Geometry check sheet. Reference: the model listing, model coordinates, mm. A direction names the side the tool comes from. Give positions to 0.01 mm unless a question says otherwise; leave off trailing zeros. Write each loop counter-clockwise with the first axis right and the second up, starting at its lowest first coordinate (ties: lowest second). Pieces come first, ordered by that corner, then holes. Notation, with made-up numbers: (72, 20.25) - (127, 20.25) arc R31 cw to (127, 45.25) - close; hole circle Ø11 at (22, -10.75). An arc over 180 degrees is marked (long way). One line per question, with ' | ' between items. Start each with the question number.
Q1. Release check for a two-part mould opening along X. For faces 1 (the face through (1.802, -72.712, 5.723)), 2 (the face through (4, -219, -4)), 3 (the face through (-209.84, 50.49, 160.9)) record: +X half, -X half, draft (parallel to the pull), parting line (faces both ways), or undercut.
Q2. Thickness scan on L1, parallel to X at y = -75.5, z = 0; L2, parallel to X at y = -131, z = 0; L3, parallel to X at y = 31, z = 112. Record the ranges inside material, lowest first. Write a range as [from, to].
Q3. Section check A-A on y = -139. Record the boundary of the cut face in (x, z), and give its area (3 significant figures).
Q4. Gauge pin test, flat ends, axial feed: P1, Ø6, axis at x = -88.5, y = -6, coming from the -Z side; P2, Ø10, axis at x = 107, z = 54.5, coming from the -Y side; P3, Ø1.5, axis at x = -139, y = -86, coming from the -Z side. Record the tip position at first contact, or that the pin passes through.
Q5. Set-up check for faces 4 (the face through (1.802, -209.321, 5.723)), 5 (the face through (-4, 50, 55)), 6 (the face through (-4, 51, 55)): record each of +Z, -Z, +X, -X, +Y, -Y from which the full face is reachable in a straight line by a thin tool's end or side.
```python
from build123d import *

# Parameters (mm, degrees)
FILLET1_R           = 20
SHELL1_T            = -1
SKETCH3_R           = 264.42717426
BOSS_EXTRUDE1_DEPTH = 1
SKETCH4_R           = 5
CUT_EXTRUDE1_DEPTH  = 451.38257191
SKETCH6_R           = 6
SKETCH6_R_2         = 5
BOSS_EXTRUDE2_DEPTH = 270
FILLET2_R           = 1


with BuildPart() as part:
    # Sketch2 → Revolve1 (revolve)
    with BuildSketch(Plane.XY):
        with BuildLine():
            Line((0, 50), (0, -200))
            ThreePointArc((0, -200), (141.421356237, -141.421356237), (200, 0))
            ThreePointArc((200, 0), (233.555453903, 23.270946312), (264.42717426, 50))
            Line((264.42717426, 50), (0, 50))
        make_face()
    revolve(axis=Axis((0, 50, 0), (0, -1, 0)))

    # Fillet1
    fillet1_edges = [part.edges().sort_by_distance(p)[0] for p in [
        (-200, 0, 0),
    ]]
    fillet(fillet1_edges, radius=FILLET1_R)

    # Shell1
    shell1_openings = [part.faces().sort_by_distance(p)[0] for p in [
        (0, 50, 0),
    ]]
    offset(amount=SHELL1_T, openings=shell1_openings, kind=Kind.INTERSECTION)

    # Sketch3 → Boss-Extrude1 (add)
    with BuildSketch(Plane(origin=(0, 50, 0), x_dir=(1, 0, 0), z_dir=(0, 1, 0))):
        Circle(SKETCH3_R)
    extrude(amount=BOSS_EXTRUDE1_DEPTH)

    # Sketch4 → Cut-Extrude1 (cut, through all)
    with BuildSketch(Plane(origin=(0, 51, 0), x_dir=(1, 0, 0), z_dir=(0, 1, 0))):
        with Locations(Location((0, 0, 0), (0, 0, 270))):
            Circle(SKETCH4_R)
    extrude(amount=-CUT_EXTRUDE1_DEPTH, mode=Mode.SUBTRACT)

    # Sketch6 → Boss-Extrude2 (add)
    with BuildSketch(Plane(origin=(0, 51, 0), x_dir=(1, 0, 0), z_dir=(0, 1, 0))):
        with Locations(Location((0, 0, 0), (0, 0, 270))):
            Circle(SKETCH6_R)
        with Locations(Location((0, 0, 0), (0, 0, 270))):
            Circle(SKETCH6_R_2, mode=Mode.SUBTRACT)
    extrude(amount=-BOSS_EXTRUDE2_DEPTH)

    # Fillet2
    fillet2_edges = [part.edges().sort_by_distance(p)[0] for p in [
        (0, 51, -5),
    ]]
    fillet(fillet2_edges, radius=FILLET2_R)


solid = part.part
```
Working result:
1) face 1: undercut | face 2: draft | face 3: parting line
2) L1: x = [-185.2, -184.12], [-6, -5], [5, 6], [184.12, 185.2] | L2: x = [-151.13, -149.8], [-6, -5], [5, 6], [149.8, 151.13] | L3: x = [-215.86, -214.09], [214.09, 215.86]
3) outline: circle Ø287.6 at (0, 0); circle Ø12 at (0, 0); hole circle Ø284.82 at (0, 0); hole circle Ø10 at (0, 0) | area: 1,290 mm2
4) P1: stops at z = -181.6 | P2: stops at y = -163.57 | P3: stops at z = -116.31
5) face 4: -Y | face 5: none | face 6: +Z, -Z, +X, -X, +Y
